Input: part model. Units: mm. Frame: model coordinates. A direction names the side the tool comes from. Give positions to 0.01 mm unless a question says otherwise; leave off trailing zeros. Loops run counter-clockwise (first coordinate to the right, second up) from the corner with the lowest first, then second, coordinate; pieces in that order, holes last. Notation, with made-up numbers: (-8.75, 27.5) - (46.25, 27.5) arc R21 ccw to (46.25, 46.5) - close; hole circle Ø5 at (3.25, 6). An arc over 180 degrees is marked (long way). One line per item, written item: value.
from build123d import *

# Parameters (mm, degrees)
BOSS_EXTRUDE1_DEPTH = 10


with BuildPart() as part:
    # Sketch1 → Boss-Extrude1 (new body)
    with BuildSketch(Plane(origin=(0, 0, 0), x_dir=(1, 0, 0), z_dir=(0, 1, 0))):
        with BuildLine():
            Line((0.566637938, 22.592895375), (128.116406017, 19.39390134))
            ThreePointArc((128.116406017, 19.39390134), (147.03, 0), (128.116406017, -19.39390134))
            Line((128.116406017, -19.39390134), (0.566637938, -22.592895375))
            ThreePointArc((0.566637938, -22.592895375), (-22.6, 0), (0.566637938, 22.592895375))
        make_face()
        with BuildLine():
            Line((0.541565463, 21.593209739), (128.091333542, 18.394215704))
            ThreePointArc((128.091333542, 18.394215704), (146.03, 0), (128.091333542, -18.394215704))
            Line((128.091333542, -18.394215704), (0.541565463, -21.593209739))
            ThreePointArc((0.541565463, -21.593209739), (-21.6, 0), (0.541565463, 21.593209739))
        make_face(mode=Mode.SUBTRACT)
    extrude(amount=BOSS_EXTRUDE1_DEPTH)


solid = part.part
Item 1: Access query for faces 1 (the face through (147.025, 4.93, -0.42)), 2 (the face through (-21.595, 4.93, 0.483)). Directions: +Z, -Z, +X, -X, +Y, -Y. A direction counts if a zero-diameter tool reaches every point of the face in a straight line with its end or side. Return the directions, or none.
Verdict:
face 1: +X, +Y, -Y
face 2: +Y, -Y
Item 2: Section B-B, the plane y = 5.25. Output: boundary loops of the cut face in (x, z), and give its area (3 significant figures).
Verdict:
outline: (0.57, -22.59) - (128.12, -19.39) arc R19.4 ccw to (128.12, 19.39) - (0.57, 22.59) arc R22.6 ccw (long way) to start; hole (0.54, -21.59) - (128.09, -18.39) arc R18.4 ccw to (128.09, 18.39) - (0.54, 21.59) arc R21.6 ccw (long way) to start
area: 384 mm^2
Item 3: Material intervals for L1, parallel to X at y = 8, z = 0; L2, parallel to Z at x = 47.5, y = 9.5; L3, parallel to X at y = 8.75, z = 17, sorted ascending.
Verdict:
L1: x = -22.6 to -21.6, 146.03 to 147.03
L2: z = -21.42 to -20.42, 20.42 to 21.42
L3: x = -14.89 to -13.33, 134.67 to 136.98
Item 4: Section A-A, the plane z = 0. Output: boundary loops of the cut face in (x, y).
Verdict:
outline: (-22.6, 0) - (-21.6, 0) - (-21.6, 10) - (-22.6, 10) - close; (146.03, 0) - (147.03, 0) - (147.03, 10) - (146.03, 10) - close
Item 5: Section C-C, the plane x = -3. Output: boundary loops of the cut face in (y, z), and give its area (3 significant figures).
Verdict:
outline: (0, -22.4) - (10, -22.4) - (10, -21.39) - (0, -21.39) - close; (0, 21.39) - (10, 21.39) - (10, 22.4) - (0, 22.4) - close
area: 20.2 mm^2
Item 6: Pin query (flat end, axial travel): P1, Ø1.5, axis at x = 94, y = 8.5, coming from the -Z side; P2, Ø6, axis at x = 20, y = 6.5, coming from the +Z side; P3, Ø1, axis at y = 5, z = 0.5, coming from the -X side. Return the tip coordinate at first contact, or that it passes through.
Verdict:
P1: stops at z = -20.27
P2: stops at z = 22.18
P3: stops at x = -22.6
Item 7: Draft query along Z for faces 3 (the face through (146.026, 4.93, -0.398)), 4 (the face through (62.6, 0, -20.2)), 5 (the face through (-22.594, 4.93, 0.505)). Return one class per face: pulls with the +Z half, pulls with the -Z half, needs draft (parallel to the pull), parting line crosses it, or undercut.
Verdict:
face 3: undercut
face 4: needs draft
face 5: parting line crosses it
